Geometry: final body of the model. Coordinates: model frame, mm. A direction names the side the tool comes from. Round coordinates to 2 decimals unless told otherwise and drop trailing zeros. Write each loop counter-clockwise with the first axis right and the second up, starting at its lowest first coordinate (ties: lowest second). Pieces come first, ordered by that corner, then holes. Notation, with made-up numbers: M 37,74.25 L 55,74.25 A18 cw 55,104.25 Z; hole C 43,62 d7. An arc over 180 degrees is marked long. Put each result on its own line as item: value. Start each with the question number.
```python
from build123d import *

# Parameters (mm, degrees)
BOSS_EXTRUDE1_DEPTH = 3.5
SKETCH8_R           = 1.5
CUT_EXTRUDE7_DEPTH  = 69.663139721
SKETCH9_R           = 3
CUT_EXTRUDE8_DEPTH  = 7
SKETCH10_R          = 7
CUT_EXTRUDE9_DEPTH  = 4.5000001
SKETCH10_3_R        = 7
CUT_EXTRUDE10_DEPTH = 4.5000001
SKETCH11_R          = 3.5
CUT_EXTRUDE11_DEPTH = 2
SKETCH12_R          = 1.5
CUT_EXTRUDE12_DEPTH = 2.5000001
SKETCH13_R          = 3.5
BOSS_EXTRUDE3_DEPTH = 1.8
SKETCH14_R          = 1.5
CUT_EXTRUDE13_DEPTH = 6.3000001
FILLET1_R           = 0.5


with BuildPart() as part:
    # Sketch1 → Boss-Extrude1 (new body, symmetric)
    with BuildSketch(Plane.XY):
        with BuildLine():
            ThreePointArc((-31.6, 0), (0, -31.6), (31.6, 0))
            ThreePointArc((31.6, 0), (37.1, 5.5), (42.6, 0))
            ThreePointArc((42.6, 0), (0, -42.6), (-42.6, 0))
            ThreePointArc((-42.6, 0), (-37.1, 5.5), (-31.6, 0))
        make_face()
    extrude(amount=BOSS_EXTRUDE1_DEPTH, both=True)

    # Sketch8 → Cut-Extrude7 (cut, through all)
    with BuildSketch(Plane(origin=(-21.3, -36.892682201, 0), x_dir=(-0.866025404, 0.5, 0), z_dir=(-0.5, -0.866025404, 0))):
        Circle(SKETCH8_R)
    cut_extrude7 = extrude(amount=-CUT_EXTRUDE7_DEPTH, mode=Mode.SUBTRACT)

    # Sketch9 → Cut-Extrude8 (cut)
    with BuildSketch(Plane(origin=(-21.3, -36.892682201, 0), x_dir=(-0.866025404, 0.5, 0), z_dir=(-0.5, -0.866025404, 0))):
        Circle(SKETCH9_R)
    cut_extrude8 = extrude(amount=-CUT_EXTRUDE8_DEPTH, mode=Mode.SUBTRACT)

    # Mirror1: Cut-Extrude7, Cut-Extrude8 across plane
    add(cut_extrude7.mirror(Plane(origin=(0, 0, 0), x_dir=(0, 0, 1), z_dir=(1, 0, 0))), mode=Mode.SUBTRACT)
    add(cut_extrude8.mirror(Plane(origin=(0, 0, 0), x_dir=(0, 0, 1), z_dir=(1, 0, 0))), mode=Mode.SUBTRACT)

    # Sketch10 → Cut-Extrude9 (cut, through all)
    with BuildSketch(Plane.XY):
        with Locations((-37.1, 0)):
            Circle(SKETCH10_R)
    extrude(amount=CUT_EXTRUDE9_DEPTH, mode=Mode.SUBTRACT)

    # Sketch10_3 → Cut-Extrude10 (cut, through all)
    with BuildSketch(Plane.XY):
        with Locations((37.1, 0)):
            Circle(SKETCH10_3_R)
    extrude(amount=-CUT_EXTRUDE10_DEPTH, mode=Mode.SUBTRACT)

    # Sketch11 → Cut-Extrude11 (cut)
    with BuildSketch(Plane.XY):
        with Locations((-37.1, 0)):
            Circle(SKETCH11_R)
    extrude(amount=-CUT_EXTRUDE11_DEPTH, mode=Mode.SUBTRACT)

    # Sketch12 → Cut-Extrude12 (cut, through all)
    with BuildSketch(Plane.XY.offset(-2)):
        with Locations((-37.1, 0)):
            Circle(SKETCH12_R)
    extrude(amount=-CUT_EXTRUDE12_DEPTH, mode=Mode.SUBTRACT)

    # Sketch13 → Boss-Extrude3 (add)
    with BuildSketch(Plane(origin=(0, 0, 0), x_dir=(-1, 0, 0), z_dir=(0, 0, -1))):
        with Locations((-37.1, 0)):
            Circle(SKETCH13_R)
    extrude(amount=BOSS_EXTRUDE3_DEPTH)

    # Sketch14 → Cut-Extrude13 (cut, through all)
    with BuildSketch(Plane(origin=(0, 0, -1.8), x_dir=(-1, 0, 0), z_dir=(0, 0, -1))):
        with Locations((-37.1, 0)):
            Circle(SKETCH14_R)
    extrude(amount=-CUT_EXTRUDE13_DEPTH, mode=Mode.SUBTRACT)

    # Fillet1
    fillet1_edges = [part.edges().sort_by_distance(p)[0] for p in [
        (40.6, 0, -1.8),
    ]]
    fillet(fillet1_edges, radius=FILLET1_R)


solid = part.part
```
1) Draft query along Z for faces 1 (the face through (35.6, -3.4, 0)), 2 (the face through (-35.8, -3.44, 0)), 3 (the face through (-18.918, -30.185, 1.291)), 4 (the face through (-35.67, 0.45, -2.74)). Return one class per face: +Z half, -Z half, draft (parallel to the pull), parting line (faces both ways), or undercut.
2) Ray query, probe 1 along X at (y, z) = (-5, 1.25); probe 2 along Y at (x, z) = (-37.1, -1.4); probe 3 along X at (y, z) = (-13.5, -0.5). Return the intervals inside material, ascending.
3) Section A-A, the plane x = -37.1. Output: boundary loops of the cut face in (y, z), and give its area (3 significant figures).
4) Section C-C, the plane x = 0. Output: boundary loops of the cut face in (y, z).
5) Section D-D, the plane x = -11.5. Output: boundary loops of the cut face in (y, z).
6) Section B-B, the plane x = 37.1. Output: boundary loops of the cut face in (y, z), and give its area (3 significant figures).
7) Access query for faces 5 (the face through (18.918, -30.185, 1.291)), 6 (the face through (35.67, 0.45, 0.81)), 7 (the face through (-0.695, -31.592, 0.049)), 8 (the face through (-33.76, 1.05, -0.99)), 9 (the face through (-37, -7, 2)). Directions: +Z, -Z, +X, -X, +Y, -Y. A direction counts if a zero-diameter tool reaches every point of the face in a straight line with its end or side. Return the directions, or none.
8) First-contact query: pin 1 (1.8 mm diameter, centred on x = 37.1, y = 0, fed in from -Z); pin 2 (6.5 mm diameter, centred on x = 36, y = 1.5, fed in from -Z); pin 3 (2 mm diameter, centred on x = -36, y = -1, fed in from +Z); pin 4 (1.5 mm diameter, centred on x = -5, z = 0, fed in from -Y). Flat tips, straight axial feed; report the tip coordinate or a pass-through.
Solved:
1. face 1: -Z half
1. face 2: +Z half
1. face 3: undercut
1. face 4: draft
2. probe 1: x = -42.31 to -42, -32.2 to -31.2, 31.2 to 42.31
2. probe 2: y = -20.94 to -3.5, 3.5 to 5.5
2. probe 3: x = -40.4 to -28.57, 28.57 to 40.4
3. outline: M -20.94,-3.5 L -1.5,-3.5 L -1.5,-2 L -3.5,-2 L -3.5,0 L -7,0 L -7,3.5 L -20.94,3.5 Z; M 1.5,-3.5 L 5.5,-3.5 L 5.5,0 L 3.5,0 L 3.5,-2 L 1.5,-2 Z
3. area: 123 mm2
4. outline: M -42.6,-3.5 L -31.6,-3.5 L -31.6,3.5 L -42.6,3.5 Z
5. outline: M -41.02,-3.5 L -29.43,-3.5 L -29.43,3.5 L -41.02,3.5 Z
6. outline: M -20.94,-3.5 L -7,-3.5 L -7,0 L -3.5,0 L -3.5,-1.3 A0.5 ccw -3,-1.8 L -1.5,-1.8 L -1.5,3.5 L -20.94,3.5 Z; M 1.5,-1.8 L 3,-1.8 A0.5 ccw 3.5,-1.3 L 3.5,0 L 5.5,0 L 5.5,3.5 L 1.5,3.5 Z
6. area: 138 mm2
7. face 5: none
7. face 6: +Z, -Z
7. face 7: +Z, -Z, +Y
7. face 8: +Z
7. face 9: +Z, +Y
8. pin 1: passes through
8. pin 2: stops at z = -1.8
8. pin 3: stops at z = -2
8. pin 4: stops at y = -42.39
